Can you work these out from the model? Positions are in its coordinate system, mm. Give positions to 0.01 mm unless a question says otherwise; leave off trailing zeros. Loops run counter-clockwise (first coordinate to the right, second up) from the corner with the lowest first, then second, coordinate; pieces in that order, holes last. Notation, with made-up numbers: (22.25, 51.5) - (66.25, 51.5) arc R21 cw to (66.25, 72.5) - close; hole circle Ø1 at (-34.5, 5). An arc over 180 degrees is marked (long way). Use a Markdown table: item, result. Add a question column.
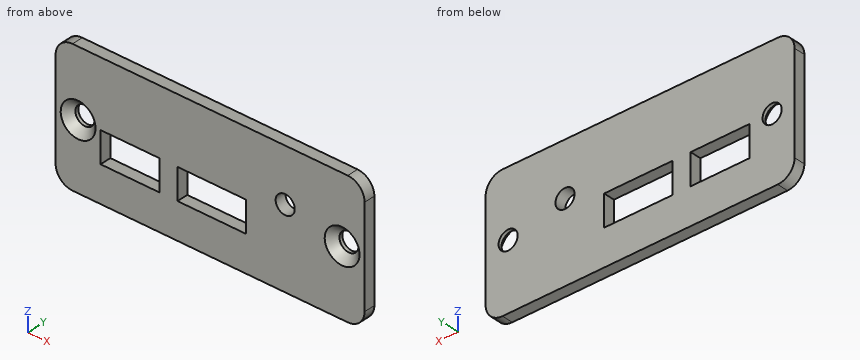
Autodesk Fusion 360 part; units mm, degrees
sketch "Skizze1" plane through (0, 0, 0) normal (0, 1, 0) x (1, 0, 0)
  line L0 (27.5, 11.8) -> (-27.5, 11.8)
  line L1 (-27.5, 11.8) -> (-27.5, -11.8)
  line L2 (-27.5, -11.8) -> (27.5, -11.8)
  line L3 (27.5, -11.8) -> (27.5, 11.8)
  line L4 (27.5, 11.8) -> (-27.5, -11.8) construction
  line L5 (-27.5, 11.8) -> (27.5, -11.8) construction
  line L6 (-19.5, -0.1) -> (-9, -0.1)
  line L7 (-9, -0.1) -> (-9, 5.4)
  line L8 (-9, 5.4) -> (-19.5, 5.4)
  line L9 (-19.5, 5.4) -> (-19.5, -0.1)
  line L10 (-5.8, -0.1) -> (6.4, -0.1)
  line L11 (6.4, -0.1) -> (6.4, 5.4)
  line L12 (6.4, 5.4) -> (-5.8, 5.4)
  line L13 (-5.8, 5.4) -> (-5.8, -0.1)
  circle A0 centre (13.3661, -2.3066) radius 1.7
  point P0 (-27.5, 0)
  point P1 (-23.5, 0)
  point P2 (23.5, 0)
  dimension "d1" = 55
  dimension "d2" = 23.6
  dimension "d3" = 10.5
  dimension "d4" = 5.5
  dimension "d5" = 5.5
  dimension "d6" = 12.2
  dimension "d7" = 3.2
  dimension "d8" = 6.4
  dimension "d9" = 8
  dimension "d10" = 3.4
  dimension "d17" = 47
  dimension "d18" = 23.5
extrude "Extrusion1" add sketch "Skizze1" along normal blind 2
hole "Bohrung1" at (23.5, 0, 0) at (-23.5, 0, 0) direction (0, 1, 0) diameter 3.4 end through all countersink diameter 6.2 countersink angle 90
fillet "Abrundung1" radius 3 4 edges at (27.5, 1, 11.8) (-27.5, 1, 11.8) (-27.5, 1, -11.8) (27.5, 1, -11.8)
equation "d5 = d4"
equation "d18 = d17 / 2"
1. Please list where these lines run through material, in increasing order: line 1 along X through (y, z) = (1.75, 0); line 2 along X through (y, z) = (0.85, -4.5); line 3 along Z through (x, y) = (0, 0.9). Write a range as [from, to].
2. Suppose I cut it at C-C (x = 23.5). List the corners of the cut face in (y, z) for me, and give its area (3 significant figures).
3. Will this pin go through, and if not, where does the flat tip stop? P1, Ø3, axis at x = 13.5, z = -6, coming from the -Y side.
4. Suppose I cut it at A-A (x = -13.5). List the corners of the cut face in (y, z) for me, and give its area (3 significant figures).
5. Suppose I cut it at B-B (y = 0.85). List the corners of the cut face in (x, z) for me, and give its area (3 significant figures).
6. Suppose I cut it at D-D (z = -2.25). State how many separate pieces and enclosed holes the cut face has, and give its area (3 significant figures).
Results below:
| question | item | result |
|---|---|---|
| 1 | line 1 | [-27.5, -25.2], [-21.8, -19.5], [-9, -5.8], [6.4, 21.8], [25.2, 27.5] |
| 1 | line 2 | [-27.5, -19.5], [-9, -5.8], [6.4, 27.5] |
| 1 | line 3 | [-11.8, -5.4], [0.1, 11.8] |
| 2 | outline | (0, -11.8) - (2, -11.8) - (2, -1.7) - (1.4, -1.7) - (0, -3.1) - close; (0, 3.1) - (1.4, 1.7) - (2, 1.7) - (2, 11.8) - (0, 11.8) - close |
| 2 | area | 38.4 mm² |
| 3 | P1 | y = 0 |
| 4 | outline | (0, -11.8) - (2, -11.8) - (2, -5.4) - (0, -5.4) - close; (0, 0.1) - (2, 0.1) - (2, 11.8) - (0, 11.8) - close |
| 4 | area | 36.2 mm² |
| 5 | outline | (-27.5, -8.8) arc R3 ccw to (-24.5, -11.8) - (24.5, -11.8) arc R3 ccw to (27.5, -8.8) - (27.5, 8.8) arc R3 ccw to (24.5, 11.8) - (-24.5, 11.8) arc R3 ccw to (-27.5, 8.8) - close; hole circle Ø4.5 at (-23.5, 0); hole (-19.5, -5.4) - (-9, -5.4) - (-9, 0.1) - (-19.5, 0.1) - close; hole (-5.8, -5.4) - (6.4, -5.4) - (6.4, 0.1) - (-5.8, 0.1) - close; hole circle Ø3.4 at (13.37, 2.31); hole circle Ø4.5 at (23.5, 0) |
| 5 | area | 1,120 mm² |
| 6 | separate pieces | 3 |
| 6 | enclosed holes | 0 |
| 6 | area | 59.9 mm² |
